from build123d import *

# Parameters (mm, degrees)
SKETCH1_R                      = 37.5
BOSS_EXTRUDE1_DEPTH            = 6
CBORE_FOR_M3_SHCS1_D           = 3.6
CBORE_FOR_M3_SHCS1_DEPTH       = 6.500114
CBORE_FOR_M3_SHCS1_CBORE_D     = 6.5
CBORE_FOR_M3_SHCS1_CBORE_DEPTH = 3
CBORE_FOR_M3_SHCS1_TIP         = 1.081549114
SKETCH7_R                      = 11.1016
CUT_EXTRUDE3_DEPTH             = 54.371340624
SKETCH8_R                      = 37.5
SKETCH8_R_2                    = 27
BOSS_EXTRUDE2_DEPTH            = 31.99999998
SKETCH5_R                      = 2.5273
CUT_EXTRUDE1_DEPTH             = 27.94
SKETCH6_R                      = 2
CUT_EXTRUDE2_DEPTH             = 60.942836102
CIRPATTERN1_COUNT              = 4
SKETCH9_R                      = 4
CUT_EXTRUDE4_DEPTH             = 24.14
CHAMFER1_SIZE                  = 0.762
CUT_EXTRUDE5_DEPTH             = 66.241857718
CUT_EXTRUDE6_START             = -29.45999998
CUT_EXTRUDE6_DEPTH             = 29.45999998
CIRPATTERN2_COUNT              = 4


with BuildPart() as part:
    # Sketch1 → Boss-Extrude1 (new body)
    with BuildSketch(Plane(origin=(0, 0, 0), x_dir=(1, 0, 0), z_dir=(0, 1, 0))):
        with Locations(Location((0, 0, 0), (0, 0, 270))):
            Circle(SKETCH1_R)
    extrude(amount=BOSS_EXTRUDE1_DEPTH)

    # CBORE for M3 SHCS1
    with Locations(Plane(origin=(0, 6, 0), x_dir=(1, 0, 0), z_dir=(0, 1, 0))):
        with Locations((-15.50195, 15.50195), (15.50195, 15.50195), (15.50195, -15.50195), (-15.50195, -15.50195)):
            CounterBoreHole(CBORE_FOR_M3_SHCS1_D / 2, CBORE_FOR_M3_SHCS1_CBORE_D / 2, CBORE_FOR_M3_SHCS1_CBORE_DEPTH, depth=CBORE_FOR_M3_SHCS1_DEPTH)
            with Locations((0, 0, -(CBORE_FOR_M3_SHCS1_DEPTH + CBORE_FOR_M3_SHCS1_TIP / 2))):  # 118° drill point
                Cone(0, CBORE_FOR_M3_SHCS1_D / 2, CBORE_FOR_M3_SHCS1_TIP, mode=Mode.SUBTRACT)

    # Sketch7 → Cut-Extrude3 (cut, through all)
    with BuildSketch(Plane(origin=(0, 6, 0), x_dir=(1, 0, 0), z_dir=(0, 1, 0))):
        with Locations(Location((0, 0, 0), (0, 0, 270))):
            Circle(SKETCH7_R)
    extrude(amount=-CUT_EXTRUDE3_DEPTH, mode=Mode.SUBTRACT)

    # Sketch8 → Boss-Extrude2 (add)
    with BuildSketch(Plane(origin=(0, 6, 0), x_dir=(1, 0, 0), z_dir=(0, 1, 0))):
        with Locations(Location((0, 0, 0), (0, 0, 270))):
            Circle(SKETCH8_R)
        with Locations(Location((0, 0, 0), (0, 0, 270))):
            Circle(SKETCH8_R_2, mode=Mode.SUBTRACT)
    extrude(amount=BOSS_EXTRUDE2_DEPTH)

    # Sketch5 → Cut-Extrude1 (cut)
    with BuildSketch(Plane(origin=(0, 0, 0), x_dir=(1, 0, 0), z_dir=(0, 1, 0))):
        with Locations(Location((0, 31.5, 0), (0, 0, 270))):
            Circle(SKETCH5_R)
    cut_extrude1 = extrude(amount=CUT_EXTRUDE1_DEPTH, mode=Mode.SUBTRACT)

    # Sketch6 → Cut-Extrude2 (cut, through all)
    with BuildSketch(Plane(origin=(0, 27.94, 0), x_dir=(-1, 0, 0), z_dir=(0, -1, 0))):
        with Locations(Location((0, 31.5, 0), (0, 0, 90))):
            Circle(SKETCH6_R)
    cut_extrude2 = extrude(amount=-CUT_EXTRUDE2_DEPTH, mode=Mode.SUBTRACT)

    # CirPattern1: Cut-Extrude1, Cut-Extrude2 ×4 about axis
    cirpattern1_axis = Axis((0, 0, 0), (0, 1, 0))
    add([cut_extrude1.rotate(cirpattern1_axis, i * 360 / CIRPATTERN1_COUNT) for i in range(1, CIRPATTERN1_COUNT)], mode=Mode.SUBTRACT)
    add([cut_extrude2.rotate(cirpattern1_axis, i * 360 / CIRPATTERN1_COUNT) for i in range(1, CIRPATTERN1_COUNT)], mode=Mode.SUBTRACT)

    # Sketch9 → Cut-Extrude4 (cut)
    with BuildSketch(Plane.XZ):
        with Locations(Location((31.5, 0, 0), (0, 0, 270))):
            Circle(SKETCH9_R)
        with Locations(Location((0, -31.5, 0), (0, 0, 270))):
            Circle(SKETCH9_R)
        with Locations(Location((-31.5, 0, 0), (0, 0, 270))):
            Circle(SKETCH9_R)
        with Locations(Location((0, 31.5, 0), (0, 0, 270))):
            Circle(SKETCH9_R)
    extrude(amount=-CUT_EXTRUDE4_DEPTH, mode=Mode.SUBTRACT)

    # Chamfer1
    chamfer1_edges = [part.edges().sort_by_distance(p)[0] for p in [
        (34.0273, 24.14, 0),
        (0, 24.14, -34.0273),
        (-34.0273, 24.14, 0),
        (0, 24.14, 34.0273),
    ]]
    chamfer(chamfer1_edges, length=CHAMFER1_SIZE)

    # Sketch10 → Cut-Extrude5 (cut, through all)
    with BuildSketch(Plane.XZ):
        with BuildLine():
            Line((-19.46, 5), (-19.46, -5))
            ThreePointArc((-19.46, -5), (-22, -7.54), (-24.54, -5))
            Line((-24.54, -5), (-24.54, 5))
            ThreePointArc((-24.54, 5), (-22, 7.54), (-19.46, 5))
        make_face()
    cut_extrude5 = extrude(amount=-CUT_EXTRUDE5_DEPTH, mode=Mode.SUBTRACT)

    # Mirror1: Cut-Extrude5 across plane
    add(cut_extrude5.mirror(Plane(origin=(0, 0, 0), x_dir=(0, 0, 1), z_dir=(1, 0, 0))), mode=Mode.SUBTRACT)

    # Sketch12 → Cut-Extrude6 (cut)
    with BuildSketch(Plane(origin=(0, 37.99999998, 0), x_dir=(1, 0, 0), z_dir=(0, 1, 0)).offset(CUT_EXTRUDE6_START)):
        with BuildLine():
            Line((-26.07999731, 6.988114218), (-36.222218486, 9.705714191))
            ThreePointArc((-36.222218486, 9.705714191), (-26.516504294, 26.516504294), (-9.705714191, 36.222218486))
            Line((-9.705714191, 36.222218486), (-6.988114218, 26.07999731))
            ThreePointArc((-6.988114218, 26.07999731), (-19.091883092, 19.091883092), (-26.07999731, 6.988114218))
        make_face()
    cut_extrude6 = extrude(amount=CUT_EXTRUDE6_DEPTH, mode=Mode.SUBTRACT)

    # CirPattern2: Cut-Extrude6 ×4 about axis
    cirpattern2_axis = Axis((0, 182.066017138, 0), (0, -1, 0))
    for i in range(1, CIRPATTERN2_COUNT):
        add(cut_extrude6.rotate(cirpattern2_axis, i * 360 / CIRPATTERN2_COUNT), mode=Mode.SUBTRACT)


solid = part.part
For this review, take the finished solid that the model builds, in its own axes (mm). A direction names the side the tool comes from. Round coordinates to 2 decimals unless told otherwise and drop trailing zeros. Loops run counter-clockwise (first coordinate to the right, second up) from the corner with the lowest first, then second, coordinate; pieces in that order, holes last. Notation, with made-up numbers: (10, 32) - (63, 32) arc R16 ccw to (63, 43) - close; hole circle Ø4 at (13.5, 82.25). An arc over 180 degrees is marked (long way). Use one line per item in the form item = value.
Item 1: Clearance check with flat-ended pins moving along their axes: P1, Ø2, axis at x = -16, z = 15, coming from the +Y side; P2, Ø7, axis at x = 17, z = 17, coming from the +Y side; P3, Ø1.5, axis at x = 2, y = 29, coming from the -Z side; P4, Ø1.8, axis at y = 2.5, z = 0, coming from the +X side. State where each tip first meets the part, or that it passes through.
Answers:
P1 = through
P2 = 8.54
P3 = -37.48
P4 = 37.5
Item 2: For line 1 (Z direction, x = 0.5, y = 4.5); line 2 (Y direction, x = -18, z = 30); line 3 (X direction, y = 3.5, z = -5.5), list the stretches that pass through material, from the lowest coordinate up.
Answers:
line_1 = -37.5 to -35.47, -27.53 to -11.09, 11.09 to 27.53, 35.47 to 37.5
line_2 = 0 to 8.54
line_3 = -37.09 to -24.49, -19.51 to -9.64, 9.64 to 19.51, 24.49 to 37.09
Item 3: Consider section B-B on x = 22. Write out the cut boundary in (y, z), then the cut area to 3 significant figures.
Answers:
outline = (0, -30.37) - (8.54, -30.37) - (8.54, -15.65) - (6, -15.65) - (6, -7.54) - (0, -7.54) - close; (0, 7.54) - (6, 7.54) - (6, 15.65) - (8.54, 15.65) - (8.54, 30.37) - (0, 30.37) - close
area = 349 mm^2
Item 4: Tool access review of faces 1 (the flat face through (-31.08, 23.064, -8.328)), 2 (the flat face through (19.46, 3, 0)), 3 (the cylindrical face through (-29.09, 26.4, -0.76)): name each direction out of +Z, -Z, +X, -X, +Y, -Y from which nothing blocks a thin tool from reaching the whole face with its end or side.
Answers:
face_1 = -Z, +Y
face_2 = +Y, -Y
face_3 = -Y
Item 5: Consider section C-C on y = 27. Write out the cut boundary in (x, z), then the cut area to 3 significant figures.
Answers:
outline = (-36.22, -9.71) - (-26.08, -6.99) arc R27 cw to (-26.08, 6.99) - (-36.22, 9.71) arc R37.5 ccw to start; (-9.71, -36.22) arc R37.5 ccw to (9.71, -36.22) - (6.99, -26.08) arc R27 cw to (-6.99, -26.08) - close; (-9.71, 36.22) - (-6.99, 26.08) arc R27 cw to (6.99, 26.08) - (9.71, 36.22) arc R37.5 ccw to start; (26.08, -6.99) - (36.22, -9.71) arc R37.5 ccw to (36.22, 9.71) - (26.08, 6.99) arc R27 cw to start; hole circle Ø5.05 at (-31.5, 0); hole circle Ø5.05 at (0, -31.5); hole circle Ø5.05 at (0, 31.5); hole circle Ø5.05 at (31.5, 0)
area = 629 mm^2
Item 6: Mouldability with a two-part tool opening along X and no side actions: class faces 4 (the flat face through (-8.366, 23.064, -31.222)), 5 (the flat face through (8.366, 23.064, 31.222)), 6 (the cylindrical face through (-33.408, 32.9, -0.601)), 7 (the cylindrical face through (-2.4, 11.9, 34.7)) as +X half, -X half, draft (parallel to the pull), parting line (faces both ways), or undercut.
Answers:
face_4 = -X half
face_5 = +X half
face_6 = undercut
face_7 = undercut
Item 7: Consider section A-A on y = 15. Write out the cut boundary in (x, z), then the cut area to 3 significant figures.
Answers:
outline = (-36.22, -9.71) - (-26.08, -6.99) arc R27 cw to (-26.08, 6.99) - (-36.22, 9.71) arc R37.5 ccw to start; (-9.71, -36.22) arc R37.5 ccw to (9.71, -36.22) - (6.99, -26.08) arc R27 cw to (-6.99, -26.08) - close; (-9.71, 36.22) - (-6.99, 26.08) arc R27 cw to (6.99, 26.08) - (9.71, 36.22) arc R37.5 ccw to start; (26.08, -6.99) - (36.22, -9.71) arc R37.5 ccw to (36.22, 9.71) - (26.08, 6.99) arc R27 cw to start; hole circle Ø8 at (-31.5, 0); hole circle Ø8 at (0, -31.5); hole circle Ø8 at (0, 31.5); hole circle Ø8 at (31.5, 0)
area = 508 mm^2
Item 8: Consider section D-D on z = 0. State how many separate pieces and enclosed holes the cut face has, then the cut area to 3 significant figures.
Answers:
separate_pieces = 6
enclosed_holes = 0
area = 422 mm^2
